```python
from build123d import *

# Parameters (mm, degrees)
ESBO_O1_W                = 40
ESBO_O1_H                = 10
RESSALTO_EXTRUS_O1_DEPTH = 1.8
CORTE_EXTRUS_O1_DEPTH    = 1.8
ESBO_O4_R                = 0.2
CORTE_EXTRUS_O2_DEPTH    = 1.8
ESBO_O5_R                = 0.2
CORTE_EXTRUS_O3_DEPTH    = 64.032052928


with BuildPart() as part:
    # Esboço1 → Ressalto-extrusão1 (new body)
    with BuildSketch(Plane.XY):
        with Locations((-37.620035336, 20.489825898)):
            Rectangle(ESBO_O1_W, ESBO_O1_H)
    extrude(amount=RESSALTO_EXTRUS_O1_DEPTH)

    # Esboço3 → Corte-extrusão1 (cut)
    with BuildSketch(Plane.XY.offset(1.8)):
        Polygon((-51.620035336, 25.489825898), (-57.620035336, 19.489825898), (-57.620035336, 25.489825898), align=None)
        Polygon((-17.620035336, 19.489825898), (-23.620035336, 25.489825898), (-17.620035336, 25.489825898), align=None)
    extrude(amount=-CORTE_EXTRUS_O1_DEPTH, mode=Mode.SUBTRACT)

    # Esboço4 → Corte-extrusão2 (cut)
    with BuildSketch(Plane.XY.offset(1.8)):
        with Locations((-41.720035336, 17.489825898)):
            Circle(ESBO_O4_R)
        with Locations((-41.720035336, 20.489825898)):
            Circle(ESBO_O4_R)
        with Locations((-41.720035336, 23.489825898)):
            Circle(ESBO_O4_R)
    extrude(amount=-CORTE_EXTRUS_O2_DEPTH, mode=Mode.SUBTRACT)

    # Esboço5 → Corte-extrusão3 (cut, through all)
    with BuildSketch(Plane.XY.offset(1.8)):
        with Locations((-53.870035336, 16.389825898)):
            Circle(ESBO_O5_R)
        with Locations((-46.370035336, 16.389825898)):
            Circle(ESBO_O5_R)
    extrude(amount=-CORTE_EXTRUS_O3_DEPTH, mode=Mode.SUBTRACT)


solid = part.part
```
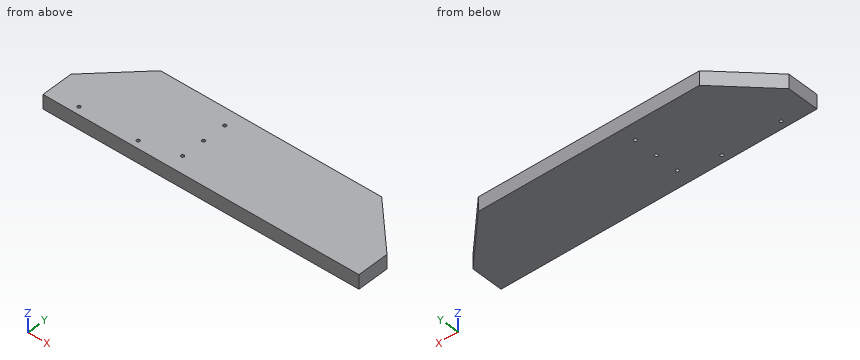
Can you work these out from the model? Positions are in its coordinate system, mm. Round coordinates to 2 decimals unless told otherwise and drop trailing zeros. Loops run counter-clockwise (first coordinate to the right, second up) from the corner with the lowest first, then second, coordinate; pieces in that order, holes last. Notation, with made-up numbers: (-38.5, 81) -> (-1.5, 81) arc R16 cw to (-1.5, 101) -> close; hole circle Ø5 at (-23, 43). An arc over 180 degrees is marked (long way). One line per item, written item: value. Start each with the question number.
1. If we section it at C-C, the plane y = 24.25: Write out the boundary of the cut face in (x, z).
2. For pin 1 (1 mm diameter, centred on x = -51.5, y = 20, fed in from -Z), with a flat end and sliding along its axis, tell me the tip position at first contact or that it passes through.
3. If I drill on probe 1 along Y at (x, z) = (-54, 0.45); probe 2 along X at (y, z) = (23, 1.6); probe 3 along X at (y, z) = (19.5, 0.8), over which ranges is the centre line in solid material (lowest first)?
4. If we section it at A-A, the plane z = 1.15: Write out the boundary of the cut face in (x, y), then the cut area to 3 significant figures.
5. If we section it at B-B, the plane x = -54.5: Write out the boundary of the cut face in (y, z), then the cut area to 3 significant figures.
Calculated:
1. outline: (-52.86, 0) -> (-22.38, 0) -> (-22.38, 1.8) -> (-52.86, 1.8) -> close
2. pin 1: stops at z = 0
3. probe 1: y = 15.49 to 16.24, 16.54 to 23.11
3. probe 2: x = -54.11 to -21.13
3. probe 3: x = -57.61 to -17.63
4. outline: (-57.62, 15.49) -> (-17.62, 15.49) -> (-17.62, 19.49) -> (-23.62, 25.49) -> (-51.62, 25.49) -> (-57.62, 19.49) -> close; hole circle Ø0.4 at (-53.87, 16.39); hole circle Ø0.4 at (-46.37, 16.39); hole circle Ø0.4 at (-41.72, 17.49); hole circle Ø0.4 at (-41.72, 20.49); hole circle Ø0.4 at (-41.72, 23.49)
4. area: 363 mm²
5. outline: (15.49, 0) -> (22.61, 0) -> (22.61, 1.8) -> (15.49, 1.8) -> close
5. area: 12.8 mm²
